Check sheet for the modelled part. Datum: model origin and axes. Units: mm. Face numbers are marked on the shaded views. Round coordinates to 2 decimals unless told otherwise and drop trailing zeros. Loops run counter-clockwise (first coordinate to the right, second up) from the corner with the lowest first, then second, coordinate; pieces in that order, holes last. Notation, with made-up numbers: (74, -23.5) -> (105, -23.5) arc R5 ccw to (105, -14.5) -> close; hole circle Ø9 at (87.5, 64.5). An arc over 180 degrees is marked (long way). Return JSON: item names as keys, results as strings.
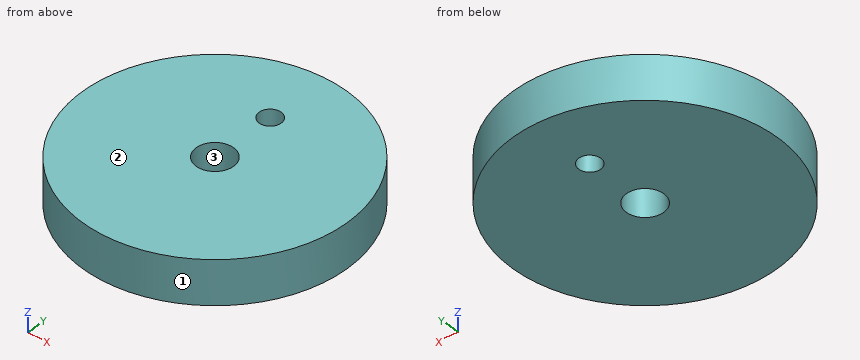
from build123d import *

# Parameters (mm, degrees)
SKETCH1_R               = 30
BOSS_EXTRUDE1_DEPTH     = 10
SKETCH2_R               = 2.5
CUT_EXTRUDE1_DEPTH      = 10
CUT_EXTRUDE4_DEPTH      = 10
CUT_EXTRUDE4_DEPTH_BACK = 10
SKETCH4_R               = 4.25


with BuildPart() as part:
    # Sketch1 → Boss-Extrude1 (new body)
    with BuildSketch(Plane.XY):
        Circle(SKETCH1_R)
    extrude(amount=BOSS_EXTRUDE1_DEPTH)

    # Sketch2 → Cut-Extrude1 (cut)
    with BuildSketch(Plane.XY):
        with Locations((0, 15)):
            Circle(SKETCH2_R)
    extrude(amount=CUT_EXTRUDE1_DEPTH, mode=Mode.SUBTRACT)

    # Sketch4 → Cut-Extrude4 (cut, two sides: drawn at the far end of the back side and taken through both)
    with BuildSketch(Plane.XY.offset(-CUT_EXTRUDE4_DEPTH_BACK)):
        Circle(SKETCH4_R)
    extrude(amount=CUT_EXTRUDE4_DEPTH + CUT_EXTRUDE4_DEPTH_BACK, mode=Mode.SUBTRACT)


solid = part.part
Q1. Section check B-B (y = 0). Record the boundary of the cut face in (x, z).
Results list:
{"outline": "(-30, 0) -> (-4.25, 0) -> (-4.25, 10) -> (-30, 10) -> close; (4.25, 0) -> (30, 0) -> (30, 10) -> (4.25, 10) -> close"}
Q2. Material ranges on line 1 (Y direction, x = 0, z = 7.25); line 2 (Y direction, x = 19.5, z = 4.5); line 3 (Y direction, x = 10, z = 4.25), recorded low to high.
Results list:
{"line 1": "-30 to -4.25, 4.25 to 12.5, 17.5 to 30", "line 2": "-22.8 to 22.8", "line 3": "-28.28 to 28.28"}
Q3. Section check D-D (y = 15). Record the boundary of the cut face in (x, z).
Results list:
{"outline": "(-25.98, 0) -> (-2.5, 0) -> (-2.5, 10) -> (-25.98, 10) -> close; (2.5, 0) -> (25.98, 0) -> (25.98, 10) -> (2.5, 10) -> close"}
Q4. Draft check along X on the marked faces 1, 2 and 3. Enter one of: released by +X, released by -X, zero draft, split by the parting line, or undercut.
Results list:
{"face 1": "split by the parting line", "face 2": "zero draft", "face 3": "undercut"}
Q5. Go/stop test with flat-tipped pins: pin 1 (6 mm diameter, centred on x = 19, z = 7.5, fed in from -Y); pin 2 (7 mm diameter, centred on x = 0, y = 0, fed in from -Z); pin 3 (1 mm diameter, centred on x = 23.5, z = 4.5, fed in from -Y); pin 4 (1 mm diameter, centred on y = -13.5, z = 8.5, fed in from -X). Record where each tip stops, or that it passes through.
Results list:
{"pin 1": "y = -25.38", "pin 2": "through", "pin 3": "y = -19.26", "pin 4": "x = -27.04"}
Q6. Section check A-A (x = 0). Record the boundary of the cut face in (y, z).
Results list:
{"outline": "(-30, 0) -> (-4.25, 0) -> (-4.25, 10) -> (-30, 10) -> close; (4.25, 0) -> (12.5, 0) -> (12.5, 10) -> (4.25, 10) -> close; (17.5, 0) -> (30, 0) -> (30, 10) -> (17.5, 10) -> close"}
Q7. Section check C-C (z = 1.25). Record the boundary of the cut face in (x, y), then the cut area to 3 significant figures.
Results list:
{"outline": "circle Ø60 at (0, 0); hole circle Ø8.5 at (0, 0); hole circle Ø5 at (0, 15)", "area": "2,750 mm^2"}
